Check sheet for the modelled part. Datum: model origin and axes. Units: mm. A direction names the side the tool comes from. Round coordinates to 2 decimals unless told otherwise and drop trailing zeros. Loops run counter-clockwise (first coordinate to the right, second up) from the corner with the lowest first, then second, coordinate; pieces in that order, holes last. Notation, with made-up numbers: (63.25, 60) -> (78.25, 60) arc R19 ccw to (78.25, 85) -> close; hole circle Ø6 at (68, -38). An arc over 180 degrees is marked (long way). One line per question, with ' | ' between items.
Autodesk Inventor part; units mm, degrees
ref_plane "YZ Plane" through (0, 0, 0) normal (1, 0, 0) x (0, 1, 0)
ref_plane "XZ Plane" through (0, 0, 0) normal (0, 1, 0) x (-1, 0, 0)
ref_plane "XY Plane" through (0, 0, 0) normal (0, 0, 1) x (1, 0, 0)
sketch "Sketch1" plane through (0, 0, 0) normal (0, 0, 1) x (1, 0, 0)
  circle A0 centre (0, 0) radius 4.125
  dimension "d0" = 8.25
extrude "Extrusion1" add sketch "Sketch1" along normal blind 77
sketch "Sketch2" plane through (0, 0, 0) normal (1, 0, 0) x (0, 1, 0)
  line L0 (-4.125, 0) -> (-4.125, 77)
  line L1 (4.125, 0) -> (4.125, 77)
  line L2 (0, -15.4) -> (0, 92.4)
  line L3 (-5.775, 0) -> (5.775, 0)
  line L4 (2.4, 0) -> (0, 0)
  line L5 (0, 5.6) -> (4.125, 5.6)
  line L6 (4.125, 5.6) -> (4.125, 0)
  line L7 (-4.125, 0) -> (-4.125, 5.6)
  line L8 (-4.125, 5.6) -> (-2.4, 0)
  line L9 (4.125, 0) -> (0, 0)
  line L10 (-2.4, 0) -> (-4.125, 0)
  point P0 (0, 3.0897)
  dimension "d4" = 5.6
revolve "Revolution1" cut sketch "Sketch2" angle 360 about axis through (0, 0, -10) along (0, 0, 1) contours L0 L8 L3
sketch "Sketch3" plane through (0, 0, 77) normal (0, 0, 1) x (1, 0, 0)
  circle A0 centre (0, 0) radius 4.125
  circle A1 centre (0, 0) radius 2.5
  dimension "d19" = 5
extrude "Extrusion2" cut sketch "Sketch3" against normal blind 42.5
sketch "Sketch4" plane through (0, 0, 34.5) normal (0, 0, 1) x (1, 0, 0)
  circle A0 centre (0, 0) radius 4.125
  circle A1 centre (0, 0) radius 3.135
  dimension "d22" = 6.27
extrude "Extrusion3" cut sketch "Sketch4" against normal blind 10
sketch "Sketch5" plane through (0, 0, 24.5) normal (0, 0, 1) x (1, 0, 0)
  circle A0 centre (0, 0) radius 4.125
  circle A1 centre (0, 0) radius 3.5
  dimension "d25" = 7
extrude "Extrusion4" cut sketch "Sketch5" against normal blind 13.5
sketch "Sketch6" plane through (0, 0, 0) normal (0, 0, -1) x (-1, 0, 0)
  circle A0 centre (0, 0) radius 2.4
  circle A1 centre (0, 0) radius 0.525
  dimension "d28" = 1.05
extrude "Extrusion5" cut sketch "Sketch6" against normal through all contours A1
properties part number "Collect_Jaw"
(1) Scan lines: probe 1 along Y at (x, z) = (0, 40) (3 decimals); probe 2 along X at (y, z) = (-0.25, 32); probe 3 along X at (y, z) = (-2, 31). Record each from-to range of solid material in increasing order.
Answer:
probe 1: y = -2.5 to -0.525, 0.525 to 2.5 | probe 2: x = -3.13 to -0.46, 0.46 to 3.13 | probe 3: x = -2.41 to 2.41
(2) Set-up check for faces 1 (the face through (2.084, 2.272, 2.217)), 2 (the face through (1.69, 2.64, 29.57)): record each of +Z, -Z, +X, -X, +Y, -Y from which the full face is reachable in a straight line by a thin tool's end or side.
Answer:
face 1: -Z | face 2: +Z
(3) Go/stop test with flat-tipped pins: pin 1 (4 mm diameter, centred on y = -2, z = 27, fed in from -X) (3 decimals); pin 2 (1.5 mm diameter, centred on x = 0.5, z = 27, fed in from +Y) (3 decimals); pin 3 (1 mm diameter, centred on x = -1.5, z = 36, fed in from -Y). Record where each tip stops, or that it passes through.
Answer:
pin 1: stops at x = -3.135 | pin 2: stops at y = 3.135 | pin 3: stops at y = -2.29
(4) Sectioned sample at A-A, the plane z = 21. Record the cut outline in (x, y) (3 decimals).
Answer:
outline: circle Ø7 at (0, 0); hole circle Ø1.05 at (0, 0)
(5) Sectioned sample at B-B, the plane z = 31. Record the cut outline in (x, y) (3 decimals), and give its area (3 significant figures).
Answer:
outline: circle Ø6.27 at (0, 0); hole circle Ø1.05 at (0, 0) | area: 30.0 mm2
